Read the model definition and answer for the solid it produces. Units are mm, in the model's axes. A direction names the side the tool comes from. Coordinates: 2 decimals unless noted, no trailing zeros. Write each loop counter-clockwise with the first axis right and the second up, starting at its lowest first coordinate (ties: lowest second). Pieces come first, ordered by that corner, then holes. Notation, with made-up numbers: M 57.25,-17.75 L 77.25,-17.75 A35 ccw 77.25,15.25 Z; hole C 23,76 d10. An arc over 180 degrees is marked long. Use a Markdown table: item, result. Add a question column.
from build123d import *

# Parameters (mm, degrees)
BOSS_EXTRUDE1_DEPTH = 100
CHAMFER1_SIZE       = 2
CHAMFER2_SIZE       = 0.5


with BuildPart() as part:
    # Sketch1 → Boss-Extrude1 (new body)
    with BuildSketch(Plane.XY):
        Polygon((50, 0), (50, 13), (-50, 13), (-50, 0), (-45.5, 0), (-45.5, 7), (45.5, 7), (45.5, 0), align=None)
    extrude(amount=BOSS_EXTRUDE1_DEPTH)

    # Chamfer1
    chamfer1_edges = [part.edges().sort_by_distance(p)[0] for p in [
        (-50, 6.5, 0),
        (50, 6.5, 100),
        (50, 6.5, 0),
        (-50, 6.5, 100),
    ]]
    chamfer(chamfer1_edges, length=CHAMFER1_SIZE)

    # Chamfer2
    chamfer2_edges = [part.edges().sort_by_distance(p)[0] for p in [
        (-50, 13, 50),
        (0, 13, 0),
        (0, 13, 100),
        (50, 13, 50),
        (-49, 13, 99),
        (49, 13, 99),
        (49, 13, 1),
        (-49, 13, 1),
    ]]
    chamfer(chamfer2_edges, length=CHAMFER2_SIZE)


solid = part.part
Item 1: This flat-tipped pin is pushed along its axis until it touches: pin 1 (1.5 mm diameter, centred on x = 20.5, z = 19.5, fed in from -Y). Where does it stop, or does it pass through?
Item 2: For faces 1 (the flat face through (-1, 7, 49)), 2 (the flat face through (-48.84, 12.75, 98.81)), determine the directions among +Z, -Z, +X, -X, +Y, -Y from which every point of the face is accessible in a straight line to the end or side of a thin tool.
Item 3: Find section B-B on z = 37. Give the vertices of the cut face in (x, y), then the cut area to 3 significant figures.
Item 4: Find section C-C on x = -18. Give the vertices of the cut face in (y, z), then the cut area to 3 significant figures.
Item 5: Consider probe 1 along X at (y, z) = (6, 47); probe 2 along Y at (x, z) = (-2.5, 87); probe 3 along Z at (x, y) = (-31, 12.75). Determine where each line is inside the solid, lowest interval first.
Item 6: Find section A-A on y = 1.5. Give the vertices of the cut face in (x, z), then the cut area to 3 significant figures.
Geometry says:
| question | item | result |
|---|---|---|
| 1 | pin 1 | stops at y = 7 |
| 2 | face 1 | +Z, -Z, -Y |
| 2 | face 2 | +Z, -X, +Y |
| 3 | outline | M -50,0 L -45.5,0 L -45.5,7 L 45.5,7 L 45.5,0 L 50,0 L 50,12.5 L 49.5,13 L -49.5,13 L -50,12.5 Z |
| 3 | area | 663 mm2 |
| 4 | outline | M 7,0 L 12.5,0 L 13,0.5 L 13,99.5 L 12.5,100 L 7,100 Z |
| 4 | area | 600 mm2 |
| 5 | probe 1 | x = -50 to -45.5, 45.5 to 50 |
| 5 | probe 2 | y = 7 to 13 |
| 5 | probe 3 | z = 0.25 to 99.75 |
| 6 | outline | M -50,2 L -48,0 L -45.5,0 L -45.5,100 L -48,100 L -50,98 Z; M 45.5,0 L 48,0 L 50,2 L 50,98 L 48,100 L 45.5,100 Z |
| 6 | area | 892 mm2 |
